```python
from build123d import *

# Parameters (mm, degrees)
PAD_DEPTH           = 10
PAD001_DEPTH        = 10
LINEARPATTERN_COUNT = 5
LINEARPATTERN_PITCH = 25
FILLET_R            = 2


with BuildPart() as part:
    # Sketch → Pad (new body)
    with BuildSketch(Plane.XY):
        Polygon((-5, 0), (-5, 120), (-10, 120), (-10, 115), (-15, 115), (-15, 125), (0, 125), (0, 0), align=None)
    extrude(amount=PAD_DEPTH)

    # Sketch001 → Pad001 (join)
    with BuildSketch(Plane.XY):
        with BuildLine():
            Line((0, 0), (0, 5))
            Line((0, 5), (7.5, 5))
            ThreePointArc((7.5, 5), (11.070714, 5.786376), (13.980741, 8))
            ThreePointArc((17.792941, 4.764706), (17.504488, 8.288453), (13.980741, 8))
            ThreePointArc((7.5, 0), (13.171134, 1.24895), (17.792941, 4.764706))
            Line((7.5, 0), (0, 0))
        make_face()
    pad001 = extrude(amount=PAD001_DEPTH)

    # LinearPattern: Pad001 ×5
    with Locations(*[(0, i * LINEARPATTERN_PITCH, 0) for i in range(1, LINEARPATTERN_COUNT)]):
        add(pad001)

    # Fillet
    fillet_edges = [part.edges().sort_by_distance(p)[0] for p in [
        (0, 125, 5),
        (-15, 125, 5),
    ]]
    fillet(fillet_edges, radius=FILLET_R)


solid = part.part
```
The listing builds one solid part. Answer for the finished solid, in the listing's coordinates (mm). A direction names the side the tool comes from. Give positions to 0.01 mm unless a question says otherwise; leave off trailing zeros. Order: outer loops, then holes, each group sorted by start corner. A loop starts at its lowest first (then second) coordinate and runs counter-clockwise, first axis right, second up. Notation, with made-up numbers: (25.5, -35) -> (55.5, -35) arc R21 cw to (55.5, 2) -> close; hole circle Ø8 at (-10.5, 34). An arc over 180 degrees is marked (long way). Answer as a JSON object with one key per item and string values. Group by question number.
Item 1: The part is cut by section A-A on x = 5. Write down the section's boundary in (y, z).
Item 2: A tool of negligible diameter and unlimited length cuts with its end or side. For faces 1 (the flat face through (-10, 118, 5)), 2 (the flat face through (4, 105, 5)), 3 (the cylindrical face through (11.024, 80.765, 4.93)), 4 (the flat face through (4, 50, 5)), from which of +Z, -Z, +X, -X, +Y, -Y can it reach the whole face along a straight path? Write none if from no direction.
Item 3: Flat-ended cylindrical pins translate along their axes: pin 1 (6 mm diameter, centred on x = 4, z = 6.5, fed in from +Y); pin 2 (1.5 mm diameter, centred on y = 85.5, z = 6, fed in from +X); pin 3 (6 mm diameter, centred on x = 5, z = 5.5, fed in from -Y); pin 4 (2 mm diameter, centred on y = 91, z = 3.5, fed in from -X). Find the tip coordinate at first contact, or state that the pin passes through.
Item 4: Consider L1, parallel to Y at x = 2, z = 2.5; L2, parallel to Y at x = 17.5, z = 4; L3, parallel to X at y = 70, z = 7.5. Determine where each line is inside the solid, lowest interval first. Write a range as from..to.
Item 5: Determine the mould class of faces 5 (the cylindrical face through (11.024, 105.765, 4.93)), 6 (the flat face through (1, 0, 5)), 7 (the flat face through (4, 75, 5)) for opening direction Y: pulls with the +Y half, pulls with the -Y half, needs draft (parallel to the pull), parting line crosses it, or undercut.
Item 6: The part is cut by section C-C on x = 11. Write down the section's boundary in (y, z), and give its area (3 significant figures).
Item 7: The part is cut by section D-D on x = -6.5. Write down the section's boundary in (y, z).
Item 8: The part is cut by section B-B on y = 46. Write down the section's boundary in (x, z), and give its area (3 significant figures).
Result set:
{
 "1": {"outline": "(0, 0) -> (5, 0) -> (5, 10) -> (0, 10) -> close; (25, 0) -> (30, 0) -> (30, 10) -> (25, 10) -> close; (50, 0) -> (55, 0) -> (55, 10) -> (50, 10) -> close; (75, 0) -> (80, 0) -> (80, 10) -> (75, 10) -> close; (100, 0) -> (105, 0) -> (105, 10) -> (100, 10) -> close"},
 "2": {"face 1": "+Z, -Z, -Y", "face 2": "+Z, -Z, +Y", "face 3": "+Z, -Z", "face 4": "+Z, -Z, +X"},
 "3": {"pin 1": "y = 105", "pin 2": "x = 0", "pin 3": "y = 0", "pin 4": "x = -5"},
 "4": {"L1": "0..5, 25..30, 50..55, 75..80, 100..105", "L2": "4.43..8.29, 29.43..33.29, 54.43..58.29, 79.43..83.29, 104.43..108.29", "L3": "-5..0"},
 "5": {"face 5": "pulls with the +Y half", "face 6": "pulls with the -Y half", "face 7": "undercut"},
 "6": {"outline": "(0.46, 0) -> (5.75, 0) -> (5.75, 10) -> (0.46, 10) -> close; (25.46, 0) -> (30.75, 0) -> (30.75, 10) -> (25.46, 10) -> close; (50.46, 0) -> (55.75, 0) -> (55.75, 10) -> (50.46, 10) -> close; (75.46, 0) -> (80.75, 0) -> (80.75, 10) -> (75.46, 10) -> close; (100.46, 0) -> (105.75, 0) -> (105.75, 10) -> (100.46, 10) -> close", "area": "265 mm²"},
 "7": {"outline": "(120, 0) -> (125, 0) -> (125, 10) -> (120, 10) -> close"},
 "8": {"outline": "(-5, 0) -> (0, 0) -> (0, 10) -> (-5, 10) -> close", "area": "50.0 mm²"}
}
